Verification items for the finished model (mm, model axes). Face numbers are marked on the shaded views. Round coordinates to 2 decimals unless told otherwise and drop trailing zeros. Loops run counter-clockwise (first coordinate to the right, second up) from the corner with the lowest first, then second, coordinate; pieces in that order, holes last. Notation, with made-up numbers: (62.5, 37.5) - (95.5, 37.5) arc R21 ccw to (95.5, 76.5) - close; hole circle Ø2 at (-14.5, -2.5). An arc over 180 degrees is marked (long way). Use a Markdown table: item, result. Add a question column.
```python
from build123d import *

# Parameters (mm, degrees)
SKETCH1_W             = 74.422
SKETCH1_H             = 50.8
BOSS_EXTRUDE1_DEPTH   = 6.35
SKETCH2_R             = 3.175
CUT_EXTRUDE1_DEPTH    = 64.289975675
SKETCH3_R             = 4.7625
CUT_EXTRUDE2_DEPTH    = 64.289975675
F_8_CLEARANCE_HOLE1_D = 4.4958
CUT_EXTRUDE3_DEPTH    = 3.175
SKETCH7_R             = 2.38125
CUT_EXTRUDE4_DEPTH    = 46.498802413
SKETCH8_R             = 0.8509
CUT_EXTRUDE5_DEPTH    = 9.525


with BuildPart() as part:
    # Sketch1 → Boss-Extrude1 (new body)
    with BuildSketch(Plane(origin=(0, 0, 0), x_dir=(1, 0, 0), z_dir=(0, 1, 0))):
        Rectangle(SKETCH1_W, SKETCH1_H)
    extrude(amount=BOSS_EXTRUDE1_DEPTH)

    # Sketch2 → Cut-Extrude1 (cut, through all)
    with BuildSketch(Plane.XY.offset(25.4)):
        with Locations((-24.511, 0)):
            Circle(SKETCH2_R)
        with Locations((26.289, 0)):
            Circle(SKETCH2_R)
    extrude(amount=-CUT_EXTRUDE1_DEPTH, mode=Mode.SUBTRACT)

    # Sketch3 → Cut-Extrude2 (cut, through all)
    with BuildSketch(Plane.XY.offset(25.4)):
        with Locations((-9.525, 0)):
            Circle(SKETCH3_R)
        with Locations((9.525, 0)):
            Circle(SKETCH3_R)
    extrude(amount=-CUT_EXTRUDE2_DEPTH, mode=Mode.SUBTRACT)

    # #8 Clearance Hole1 (through all)
    with Locations(Plane(origin=(0, 6.35, 0), x_dir=(1, 0, 0), z_dir=(0, 1, 0))):
        with Locations((-32.4485, 12.7), (-32.4485, -12.7), (-17.399, -12.7), (0, -12.7), (17.399, -12.7), (32.4485, -12.7), (32.4485, 12.7), (17.399, 12.7), (0, 12.7), (-17.399, 12.7)):
            Hole(F_8_CLEARANCE_HOLE1_D / 2)

    # Sketch6 → Cut-Extrude3 (cut)
    with BuildSketch(Plane(origin=(0, 6.35, 0), x_dir=(1, 0, 0), z_dir=(0, 1, 0))):
        with BuildLine():
            Line((-13.081, 17.018), (-13.081, 8.382))
            ThreePointArc((-13.081, 8.382), (-17.399, 4.064), (-21.717, 8.382))
            Line((-21.717, 8.382), (-21.717, 17.018))
            ThreePointArc((-21.717, 17.018), (-17.399, 21.336), (-13.081, 17.018))
        make_face()
        with BuildLine():
            Line((13.081, 17.018), (13.081, 8.382))
            ThreePointArc((13.081, 8.382), (17.399, 4.064), (21.717, 8.382))
            Line((21.717, 8.382), (21.717, 17.018))
            ThreePointArc((21.717, 17.018), (17.399, 21.336), (13.081, 17.018))
        make_face()
        with BuildLine():
            Line((13.081, -17.018), (13.081, -8.382))
            ThreePointArc((13.081, -8.382), (17.399, -4.064), (21.717, -8.382))
            Line((21.717, -8.382), (21.717, -17.018))
            ThreePointArc((21.717, -17.018), (17.399, -21.336), (13.081, -17.018))
        make_face()
        with BuildLine():
            Line((-13.081, -17.018), (-13.081, -8.382))
            ThreePointArc((-13.081, -8.382), (-17.399, -4.064), (-21.717, -8.382))
            Line((-21.717, -8.382), (-21.717, -17.018))
            ThreePointArc((-21.717, -17.018), (-17.399, -21.336), (-13.081, -17.018))
        make_face()
        with BuildLine():
            Line((4.318, 17.018), (4.318, 8.382))
            ThreePointArc((4.318, 8.382), (0, 4.064), (-4.318, 8.382))
            Line((-4.318, 8.382), (-4.318, 17.018))
            ThreePointArc((-4.318, 17.018), (0, 21.336), (4.318, 17.018))
        make_face()
        with BuildLine():
            Line((4.318, -17.018), (4.318, -8.382))
            ThreePointArc((4.318, -8.382), (0, -4.064), (-4.318, -8.382))
            Line((-4.318, -8.382), (-4.318, -17.018))
            ThreePointArc((-4.318, -17.018), (0, -21.336), (4.318, -17.018))
        make_face()
        with BuildLine():
            Line((-28.1305, 17.018), (-28.1305, 8.382))
            ThreePointArc((-28.1305, 8.382), (-32.4485, 4.064), (-36.7665, 8.382))
            Line((-36.7665, 8.382), (-36.7665, 17.018))
            ThreePointArc((-36.7665, 17.018), (-32.4485, 21.336), (-28.1305, 17.018))
        make_face()
        with BuildLine():
            Line((-28.1305, -17.018), (-28.1305, -8.382))
            ThreePointArc((-28.1305, -8.382), (-32.4485, -4.064), (-36.7665, -8.382))
            Line((-36.7665, -8.382), (-36.7665, -17.018))
            ThreePointArc((-36.7665, -17.018), (-32.4485, -21.336), (-28.1305, -17.018))
        make_face()
        with BuildLine():
            Line((28.1305, 17.018), (28.1305, 8.382))
            ThreePointArc((28.1305, 8.382), (32.4485, 4.064), (36.7665, 8.382))
            Line((36.7665, 8.382), (36.7665, 17.018))
            ThreePointArc((36.7665, 17.018), (32.4485, 21.336), (28.1305, 17.018))
        make_face()
        with BuildLine():
            Line((28.1305, -17.018), (28.1305, -8.382))
            ThreePointArc((28.1305, -8.382), (32.4485, -4.064), (36.7665, -8.382))
            Line((36.7665, -8.382), (36.7665, -17.018))
            ThreePointArc((36.7665, -17.018), (32.4485, -21.336), (28.1305, -17.018))
        make_face()
    extrude(amount=-CUT_EXTRUDE3_DEPTH, mode=Mode.SUBTRACT)

    # Sketch7 → Cut-Extrude4 (cut, through all)
    with BuildSketch(Plane(origin=(0, 6.35, 0), x_dir=(1, 0, 0), z_dir=(0, 1, 0))):
        with Locations(Location((0, 0, 0), (0, 0, 270))):
            Circle(SKETCH7_R)
    extrude(amount=-CUT_EXTRUDE4_DEPTH, mode=Mode.SUBTRACT)

    # Sketch8 → Cut-Extrude5 (cut)
    with BuildSketch(Plane.XY.offset(25.4)):
        with Locations((0, 1.5875)):
            Circle(SKETCH8_R)
    extrude(amount=-CUT_EXTRUDE5_DEPTH, mode=Mode.SUBTRACT)


solid = part.part
```
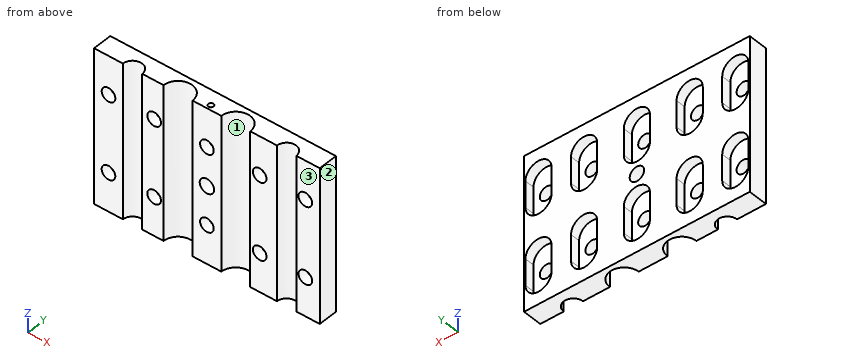
Q1. Go/stop test with flat-tipped pins: pin 1 Ø2 at (x, z) = (25.5, -18.5) entering from -Y; pin 2 Ø4.5 at (x, z) = (1.5, 8.5) entering from +Y (3 decimals). Record where each tip stops, or that it passes through.
Q2. Section check B-B on x = 0. Record the cut outline in (y, z) (3 decimals), plus the area to 3 significant figures.
Q3. Section check D-D on z = -12.7. State how many separate pieces and enclosed holes the cut face has, plus the area to 3 significant figures.
Q4. Thickness scan on line 1 along X through (y, z) = (1.5, 10); line 2 along X through (y, z) = (5.5, -21); line 3 along X through (y, z) = (5.5, 20.5). Record the ranges inside material, lowest first.
Q5. Release check for a two-part mould opening along X. For the marked faces 1, 2 and 3 record: +X half, -X half, draft (parallel to the pull), parting line (faces both ways), or undercut.
Determined:
| question | item | result |
|---|---|---|
| 1 | pin 1 | stops at y = 2.62 |
| 1 | pin 2 | stops at y = 3.175 |
| 2 | outline | (0, -25.4) - (6.35, -25.4) - (6.35, -21.336) - (3.175, -21.336) - (3.175, -14.948) - (0, -14.948) - close; (0, -10.452) - (3.175, -10.452) - (3.175, -4.064) - (6.35, -4.064) - (6.35, -2.381) - (0, -2.381) - close; (0, 2.381) - (6.35, 2.381) - (6.35, 4.064) - (3.175, 4.064) - (3.175, 10.452) - (0, 10.452) - close; (0, 14.948) - (3.175, 14.948) - (3.175, 21.336) - (6.35, 21.336) - (6.35, 25.4) - (2.438, 25.4) - (2.438, 15.875) - (0.737, 15.875) - (0.737, 25.4) - (0, 25.4) - close |
| 2 | area | 138 mm² |
| 3 | separate pieces | 6 |
| 3 | enclosed holes | 0 |
| 3 | area | 161 mm² |
| 4 | line 1 | x = -37.21 to -27.31, -21.71 to -14.05, -5 to 5, 14.05 to 23.49, 29.09 to 37.21 |
| 4 | line 2 | x = -37.21 to -34.12, -30.78 to -19.07, -15.73 to -1.67, 1.67 to 15.73, 19.07 to 30.78, 34.12 to 37.21 |
| 4 | line 3 | x = -37.21 to -35, -29.89 to -19.95, -14.85 to -2.55, 2.55 to 14.85, 19.95 to 29.89, 35 to 37.21 |
| 5 | face 1 | undercut |
| 5 | face 2 | +X half |
| 5 | face 3 | draft |
